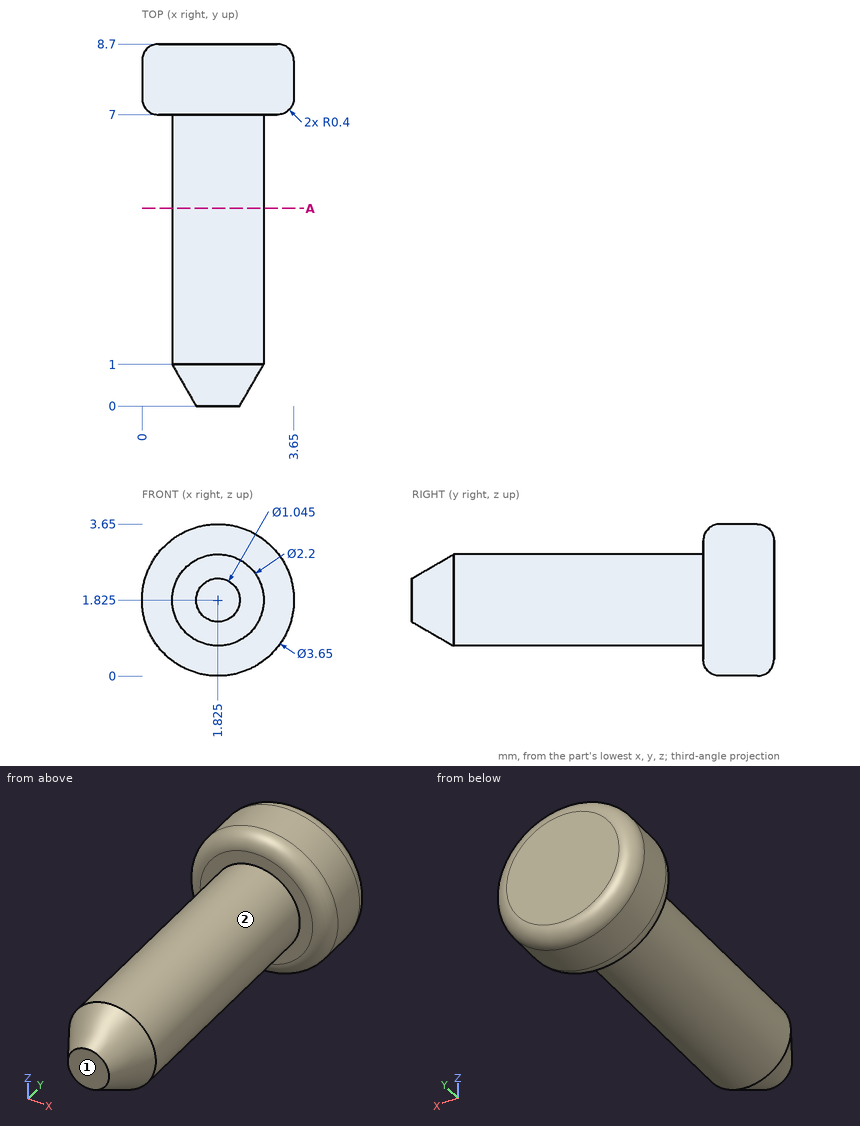
Answer from the drawing. Dimensions are ordinates in mm from the lowest x, y and z of the part. A direction names the side the tool comes from. Coordinates: 2 decimals unless noted, no trailing zeros. Loops run counter-clockwise (first coordinate to the right, second up) from the corner with the lowest first, then second, coordinate; pieces in that order, holes last. Notation, with made-up numbers: (56, -31) -> (101, -31) arc R14 ccw to (101, -6) -> close; hole circle Ø9 at (86.5, 32). An arc over 180 degrees is marked (long way). Answer in a Markdown table with one row per item.
Item 1: For the marked faces 1 and 2, determine the directions among +Z, -Z, +X, -X, +Y, -Y from which every point of the face is accessible in a straight line to the end or side of a thin tool.
Returned:
| item | result |
|---|---|
| face 1 | +Z, -Z, +X, -X, -Y |
| face 2 | -Y |
Item 2: Straight lines are drawn through the part: line 1 along Y through (x, z) = (2.1, 0.5); line 2 along X through (y, z) = (2.25, 2); line 3 along X through (y, z) = (7.5, 1.65). For each, find the intervals that lie inside material, in ascending order. Write a range as [from, to].
Returned:
| item | result |
|---|---|
| line 1 | y = [7, 8.7] |
| line 2 | x = [0.74, 2.91] |
| line 3 | x = [0.01, 3.64] |
Item 3: A cutting plane is placed at A-A on y = 4.75. Determine the outline of the cut face in (x, z) (1 decimal).
Returned:
| item | result |
|---|---|
| outline | circle Ø2.2 at (1.8, 1.8) |
Item 4: Each of these flat-tipped pins is pushed along its axis until it touches: P1, Ø2, axis at y = 3.5, z = 1, coming from the +X side (3 decimals); P2, Ø1.5, axis at x = 0.5, y = 5, coming from the +Z side. Where does it stop, or does it pass through?
Returned:
| item | result |
|---|---|
| P1 | stops at x = 2.925 |
| P2 | stops at z = 2.76 |
